Design review of the part built by this model. Coordinates are the model's own, in mm. Face numbers are marked on the shaded views. A direction names the side the tool comes from. Coordinates: 2 decimals unless noted, no trailing zeros. Order: outer loops, then holes, each group sorted by start corner. A loop starts at its lowest first (then second) coordinate and runs counter-clockwise, first axis right, second up. Notation, with made-up numbers: (43, 9) -> (59, 9) arc R30 ccw to (59, 41) -> close; hole circle Ø4 at (75.25, 49.5). An arc over 180 degrees is marked (long way). Write item = value, one per line.
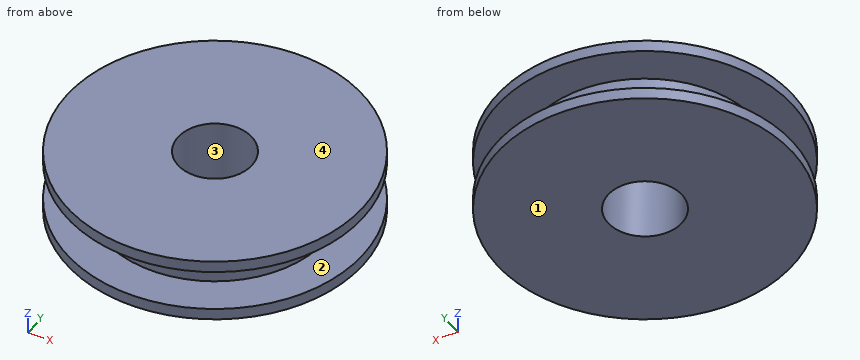
```python
from build123d import *

# Parameters (mm, degrees)
F0_R     = 12.7
F0_R_2   = 3.175
F1_DEPTH = 1.00000054
F2_R     = 9.525
F2_R_2   = 3.175
F3_DEPTH = 3.556
F4_R     = 12.7
F4_R_2   = 9.525
F4_R_3   = 3.175
F5_DEPTH = 1.00000054


# Not quite as in the source:
# - a feature names something its author has since deleted; it is built from what else it names


with BuildPart() as f1:
    # F0 (on Top) → F1 (new body)
    with BuildSketch(Plane.XY):
        Circle(F0_R)
        Circle(F0_R_2, mode=Mode.SUBTRACT)
    extrude(amount=F1_DEPTH)

    # F2 (on face) → F3 (join)
    with BuildSketch(Plane.XY.offset(1.00000054)):
        Circle(F2_R)
        Circle(F2_R_2, mode=Mode.SUBTRACT)
    extrude(amount=F3_DEPTH)

    # F4 (on face) → F5 (join)
    with BuildSketch(Plane.XY.offset(4.55600054)):
        Circle(F4_R)
        Circle(F4_R_2, mode=Mode.SUBTRACT)
        Circle(F4_R_2)
        Circle(F4_R_3, mode=Mode.SUBTRACT)
    extrude(amount=F5_DEPTH)


solid = f1.part
```
(1) We need section C-C (z = 3.25). Write out the cut boundary in (x, y) (3 decimals), and give its area (3 significant figures).
Report:
outline = circle Ø19.05 at (0, 0); hole circle Ø6.35 at (0, 0)
area = 253 mm²
(2) We need section D-D (x = 10). Write out the cut boundary in (y, z), and give its area (3 significant figures).
Report:
outline = (-7.83, 0) -> (7.83, 0) -> (7.83, 1) -> (-7.83, 1) -> close; (-7.83, 4.56) -> (7.83, 4.56) -> (7.83, 5.56) -> (-7.83, 5.56) -> close
area = 31.3 mm²
(3) The part is to be moulded in two halves that separate along X. For the marked faces 3 and 4, say which applies: released by +X, released by -X, zero draft, split by the parting line, or undercut.
Report:
face_3 = undercut
face_4 = zero draft
(4) We need section A-A (y = 0). Write out the cut boundary in (x, z) (3 decimals).
Report:
outline = (-12.7, 0) -> (-3.175, 0) -> (-3.175, 5.556) -> (-12.7, 5.556) -> (-12.7, 4.556) -> (-9.525, 4.556) -> (-9.525, 1) -> (-12.7, 1) -> close; (3.175, 0) -> (12.7, 0) -> (12.7, 1) -> (9.525, 1) -> (9.525, 4.556) -> (12.7, 4.556) -> (12.7, 5.556) -> (3.175, 5.556) -> close
(5) For the marked faces 1 and 2, list the 3-axis set-ups (+Z, -Z, +X, -X, +Y, -Y) from which the entire face can be reached by the end or side of a thin tool; tool diameter is ignored.
Report:
face_1 = -Z, +X, -X, +Y, -Y
face_2 = none
(6) Insertion check: pin 1 (3 mm diameter, centred on x = -3.5, z = 3, fed in from +Y). The pin has a flat end and moves straight along its axis. Give the tip position at first contact, or say it passes through.
Report:
pin_1 = 9.31
(7) For L1, parallel to Y at x = 0, z = 4 (3 decimals); L2, parallel to Z at x = -7, y = 6.5; L3, parallel to X at y = 2.25, z = 0.3, list the stretches that pass through material, from the lowest coordinate up.
Report:
L1 = -9.525 to -3.175, 3.175 to 9.525
L2 = 0 to 1, 4.56 to 5.56
L3 = -12.5 to -2.24, 2.24 to 12.5
